from build123d import *

# Parameters (mm, degrees)
F0_R     = 5
F1_DEPTH = 40
F2_R     = 5
F3_DEPTH = 10


with BuildPart() as f1:
    # F0 (on Top) → F1 (new body)
    with BuildSketch(Plane.XY):
        with BuildLine():
            Line((-84.020619, -2.304368), (-4.020619, -2.304368))
            Line((-4.020619, -2.304368), (-4.020619, 37.695632))
            Line((-4.020619, 37.695632), (-22.312074, 37.695632))
            ThreePointArc((-22.312074, 37.695632), (-44.020619, 15.987087), (-65.729164, 37.695632))
            Line((-65.729164, 37.695632), (-84.020619, 37.695632))
            Line((-84.020619, 37.695632), (-84.020619, -2.304368))
        make_face()
        with Locations((-74.020619, 7.695632)):
            Circle(F0_R, mode=Mode.SUBTRACT)
        with Locations((-14.020619, 7.695632)):
            Circle(F0_R, mode=Mode.SUBTRACT)
    extrude(amount=F1_DEPTH)

    # F2 (on face) → F3 (cut)
    with BuildSketch(Plane.XY.offset(40)):
        with BuildLine():
            Line((-84.020619, 22.695632), (-59.713322, 22.695632))
            ThreePointArc((-59.713322, 22.695632), (-64.169151, 29.61494), (-65.729164, 37.695632))
            Line((-65.729164, 37.695632), (-84.020619, 37.695632))
            Line((-84.020619, 37.695632), (-84.020619, 22.695632))
        make_face()
        with BuildLine():
            ThreePointArc((-22.312074, 37.695632), (-28.67036, 22.345372), (-44.020619, 15.987087))
            Line((-44.020619, 15.987087), (-44.020619, -2.304368))
            Line((-44.020619, -2.304368), (-4.020619, -2.304368))
            Line((-4.020619, -2.304368), (-4.020619, 37.695632))
            Line((-4.020619, 37.695632), (-22.312074, 37.695632))
        make_face()
        with Locations((-14.020619, 7.695632)):
            Circle(F2_R, mode=Mode.SUBTRACT)
    extrude(amount=-F3_DEPTH, mode=Mode.SUBTRACT)


solid = f1.part
CAD build for the part. Positions are in the model's coordinates, mm. A direction names the side the tool comes from. Round coordinates to 2 decimals unless told otherwise and drop trailing zeros. Write each loop counter-clockwise with the first axis right and the second up, starting at its lowest first coordinate (ties: lowest second). Pieces come first, ordered by that corner, then holes. Notation, with made-up numbers: M -29,-7.5 L -1,-7.5 A17 cw -1,-3.5 Z; hole C 17.25,-30 d7. An arc over 180 degrees is marked long. Put each result on its own line as item: value. Start each with the question number.
1) 3-axis set-ups, long thin cutter, end or side, ignore diameter. For faces 1 (the flat face through (-13, 37.696, 15)), 2 (the flat face through (-75, 30, 30)), 3 (the flat face through (-44.021, 7, 35)): which of +Z, -Z, +X, -X, +Y, -Y reach the whole face in a straight line?
2) Pull direction Y, two halves, no side cores. Call faces 4 (the cylindrical face through (-69.252, 9.197, 19.72)), 5 (the cylindrical face through (-9.252, 9.197, 14.79)), 6 (the flat face through (-20, 14, 30)), 7 (the flat face through (-72, 22.696, 35)): pulls with the +Y half, pulls with the -Y half, needs draft (parallel to the pull), parting line crosses it, or undercut.
3) Drill centre lines: probe 1 along X at (y, z) = (10.5, 27); probe 2 along Y at (x, z) = (-74, 9.5); probe 3 along Y at (x, z) = (-72, 5.5). Where is each one in solid material? Low to high. Write a range as [from, to].
4) Saw through at A-A, the plane y = 34. Write the cut outline in (x, z), and give its area (3 significant figures).
5) Saw through at D-D, the plane x = -75. Write the cut outline in (y, z).
6) Saw through at C-C, the plane z = 26.5. Write the cut outline in (x, y).
7) Pin check, flat tips, straight feed: pin 1 Ø8 at (x, y) = (-21.5, 7) entering from -Z; pin 2 Ø5 at (x, z) = (-71, 34.5) entering from +Y; pin 3 Ø5 at (y, z) = (10.5, 37.5) entering from +X; pin 4 Ø4.5 at (x, y) = (-75, 31.5) entering from +Z. Stop position of each tip, or through.
8) Saw through at B-B, the plane y = 9.5. Write the cut outline in (x, z), and give its area (3 significant figures).
Resolved:
1. face 1: +Z, -Z, +X, -X, +Y
1. face 2: +Z, +X, -X, +Y
1. face 3: +Z, +X, +Y, -Y
2. face 4: undercut
2. face 5: undercut
2. face 6: needs draft
2. face 7: pulls with the +Y half
3. probe 1: [-84.02, -78.16], [-69.88, -18.16], [-9.88, -4.02]
3. probe 2: [-2.3, 2.7], [12.7, 37.7]
3. probe 3: [-2.3, 3.12], [12.27, 37.7]
4. outline: M -84.02,0 L -65.41,0 L -65.41,30 L -84.02,30 Z; M -22.63,0 L -4.02,0 L -4.02,30 L -22.63,30 Z
4. area: 1,120 mm²
5. outline: M -2.3,0 L 2.79,0 L 2.79,40 L -2.3,40 Z; M 12.6,0 L 37.7,0 L 37.7,30 L 22.7,30 L 22.7,40 L 12.6,40 Z
6. outline: M -84.02,-2.3 L -4.02,-2.3 L -4.02,37.7 L -22.31,37.7 A21.71 cw -65.73,37.7 L -84.02,37.7 Z; hole C -74.02,7.7 d10; hole C -14.02,7.7 d10
7. pin 1: z = 0
7. pin 2: y = 22.7
7. pin 3: x = -44.02
7. pin 4: z = 30
8. outline: M -84.02,0 L -78.68,0 L -78.68,40 L -84.02,40 Z; M -69.36,0 L -18.68,0 L -18.68,30 L -44.02,30 L -44.02,40 L -69.36,40 Z; M -9.36,0 L -4.02,0 L -4.02,30 L -9.36,30 Z
8. area: 2,150 mm²
